from build123d import *

# Parameters (mm, degrees)
EXTRUDE_1_DEPTH     = 13.6
SKETCH_3_W          = 16
SKETCH_3_H          = 7.9
CUT_EXTRUDE_3_DEPTH = 1
SKETCH_5_W          = 21
SKETCH_5_H          = 16
EXTRUDE_2_DEPTH     = 6
SKETCH_5_4_W        = 17
SKETCH_5_4_H        = 16
EXTRUDE_3_DEPTH     = 7.7


with BuildPart() as part:
    # Эскиз1 → Бобышка-Вытянуть1 (new body)
    with BuildSketch(Plane(origin=(0, 0, 0), x_dir=(1, 0, 0), z_dir=(0, 1, 0))):
        with BuildLine():
            Line((41, 31), (-41, 31))
            ThreePointArc((-41, 31), (-44.535533906, 29.535533906), (-46, 26))
            Line((-46, 26), (-46, -26))
            ThreePointArc((-46, -26), (-44.535533906, -29.535533906), (-41, -31))
            Line((-41, -31), (41, -31))
            ThreePointArc((41, -31), (44.535533906, -29.535533906), (46, -26))
            Line((46, -26), (46, 26))
            ThreePointArc((46, 26), (44.535533906, 29.535533906), (41, 31))
        make_face()
    extrude(amount=EXTRUDE_1_DEPTH)

    # Эскиз3 → Вырез-Вытянуть3 (cut)
    with BuildSketch(Plane(origin=(46, 0, 0), x_dir=(0, 0, -1), z_dir=(1, 0, 0))):
        with Locations((-18, 9.65)):
            Rectangle(SKETCH_3_W, SKETCH_3_H)
        with Locations((0.5, 9.65)):
            Rectangle(SKETCH_3_W, SKETCH_3_H)
        with Locations((19, 9.65)):
            Rectangle(SKETCH_3_W, SKETCH_3_H)
    extrude(amount=-CUT_EXTRUDE_3_DEPTH, mode=Mode.SUBTRACT)

    # Эскиз5 → Бобышка-Вытянуть2 (add)
    with BuildSketch(Plane(origin=(0, 13.6, 0), x_dir=(1, 0, 0), z_dir=(0, 1, 0))):
        with Locations((34.5, -18)):
            Rectangle(SKETCH_5_W, SKETCH_5_H)
    extrude(amount=EXTRUDE_2_DEPTH)

    # Эскиз5<4> → Бобышка-Вытянуть3 (add)
    with BuildSketch(Plane(origin=(0, 13.6, 0), x_dir=(1, 0, 0), z_dir=(0, 1, 0))):
        with Locations((36.5, 0.5)):
            Rectangle(SKETCH_5_4_W, SKETCH_5_4_H)
        with Locations((36.5, 19)):
            Rectangle(SKETCH_5_4_W, SKETCH_5_4_H)
    extrude(amount=EXTRUDE_3_DEPTH)


solid = part.part
Part model, mm, in its own coordinate system. A direction names the side the tool comes from. Round coordinates to 2 decimals unless told otherwise and drop trailing zeros. Loops run counter-clockwise (first coordinate to the right, second up) from the corner with the lowest first, then second, coordinate; pieces in that order, holes last. Notation, with made-up numbers: (-16, -10.75) - (-4, -10.75) arc R13 ccw to (-4, -3.75) - close; hole circle Ø4 at (62, 23). An arc over 180 degrees is marked (long way). Answer as a JSON object with one key per item and string values.
Item 1: Band-saw the part on C-C on z = -1. List the corners of the cut face in (x, y).
Output:
{"outline": "(-46, 0) - (46, 0) - (46, 5.7) - (45, 5.7) - (45, 21.3) - (28, 21.3) - (28, 13.6) - (-46, 13.6) - close"}
Item 2: Band-saw the part on D-D on x = 8.5. List the corners of the cut face in (y, z).
Output:
{"outline": "(0, -31) - (13.6, -31) - (13.6, 31) - (0, 31) - close"}
Item 3: Band-saw the part on A-A on x = 29.5. List the corners of the cut face in (y, z), plus the area to 3 significant figures.
Output:
{"outline": "(0, -31) - (13.6, -31) - (13.6, -27) - (21.3, -27) - (21.3, -11) - (13.6, -11) - (13.6, -8.5) - (21.3, -8.5) - (21.3, 7.5) - (13.6, 7.5) - (13.6, 10) - (19.6, 10) - (19.6, 26) - (13.6, 26) - (13.6, 31) - (0, 31) - close", "area": "1,190 mm2"}
Item 4: Tool access for faces 5 (the face through (36, 17, -27)), 6 (the face through (28, 17, 0)), 7 (the face through (45, 14, -19)): list every direction of +Z, -Z, +X, -X, +Y, -Y with a clear straight run to the whole face (end or side of a thin tool).
Output:
{"face 5": "-Z, +X, -X, +Y", "face 6": "-Z, -X, +Y", "face 7": "+X, +Y"}
Item 5: Pull direction Z, two halves, no side cores. Call faces 1 (the face through (45, 13, 18)), 2 (the face through (46, 2, 0)), 3 (the face through (-45, 7, 29)), 4 (the face through (36, 17, -8.5)): pulls with the +Z half, pulls with the -Z half, needs draft (parallel to the pull), parting line crosses it, or undercut.
Output:
{"face 1": "undercut", "face 2": "needs draft", "face 3": "pulls with the +Z half", "face 4": "undercut"}
Item 6: Wall check: L1, parallel to Z at x = 31, y = 18; L2, parallel to X at y = 8, z = -1.5; L3, parallel to X at y = 14, z = -12. Give the ranges that are in metal, low to high.
Output:
{"L1": "-27 to -11, -8.5 to 7.5, 10 to 26", "L2": "-46 to 45", "L3": "28 to 45"}
Item 7: Pin check, flat tips, straight feed: pin 1 (4 mm diameter, centred on y = 19, z = -1.5, fed in from -X); pin 2 (1 mm diameter, centred on x = 13.5, z = 1.5, fed in from +Y); pin 3 (1.8 mm diameter, centred on x = 34.5, y = 16, fed in from -Z); pin 4 (1.5 mm diameter, centred on x = -8.5, y = 15, fed in from -Z). Stop position of each tip, or through.
Output:
{"pin 1": "x = 28", "pin 2": "y = 13.6", "pin 3": "z = -27", "pin 4": "through"}
Item 8: Band-saw the part on B-B on z = 11.5. List the corners of the cut face in (x, y).
Output:
{"outline": "(-46, 0) - (46, 0) - (46, 5.7) - (45, 5.7) - (45, 19.6) - (24, 19.6) - (24, 13.6) - (-46, 13.6) - close"}
